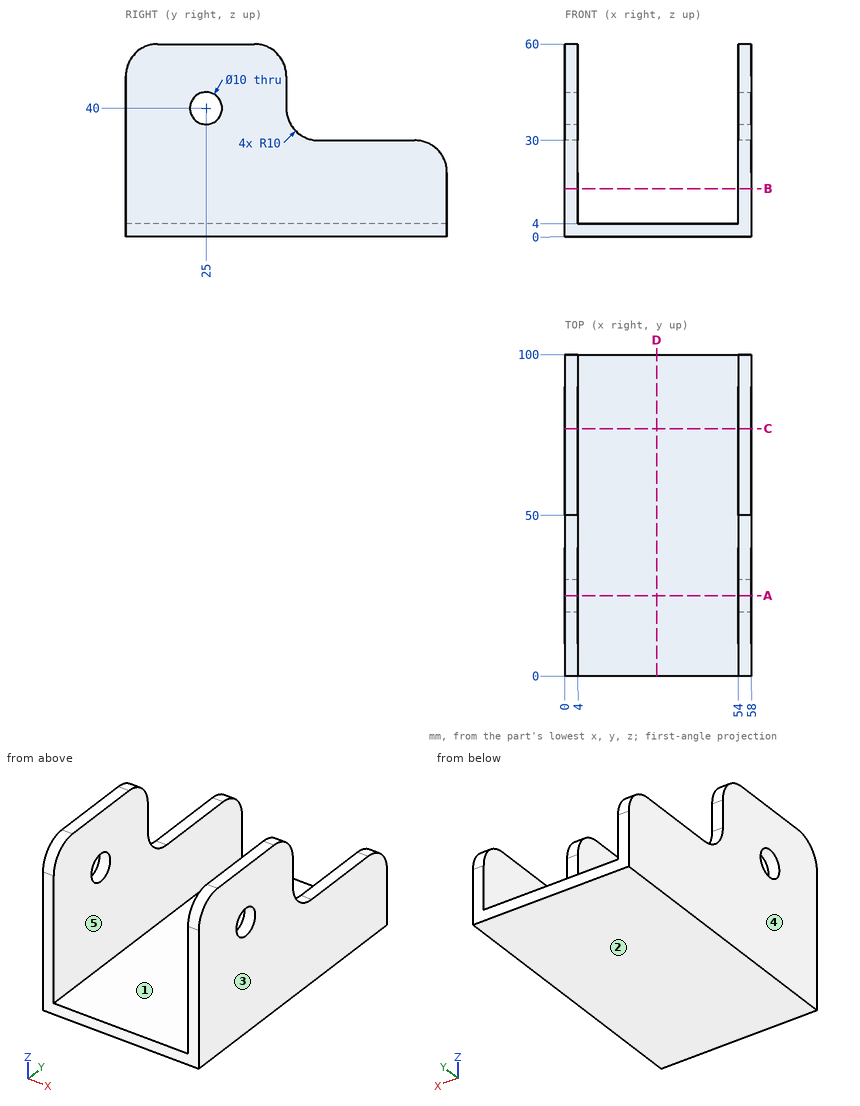
Verification items for this drawing (mm, ordinates from the low corner). A direction names the side the tool comes from. Round coordinates to 2 decimals unless told otherwise and drop trailing zeros. Order: outer loops, then holes, each group sorted by start corner. A loop starts at its lowest first (then second) coordinate and runs counter-clockwise, first axis right, second up. Notation, with made-up numbers: (4.25, 89.25) -> (11.25, 89.25) arc R28 cw to (11.25, 119.25) -> close; hole circle Ø9 at (0, 46). An arc over 180 degrees is marked (long way). Use one line per item in the form item = value.
1. Cross-section at C-C, the plane y = 77. Enter the section's corners in (x, z).
Working result:
outline = (0, 0) -> (58, 0) -> (58, 30) -> (54, 30) -> (54, 4) -> (4, 4) -> (4, 30) -> (0, 30) -> close
2. Scan lines: line 1 along Z through (x, y) = (1, 25); line 2 along X through (y, z) = (80.5, 13.5); line 3 along Z through (x, y) = (2, 67.5). Record each from-to range of solid material in increasing order. Write a range as from..to.
Working result:
line_1 = 0..35, 45..60
line_2 = 0..4, 54..58
line_3 = 0..30
3. Cross-section at D-D, the plane x = 28.5. Enter the section's corners in (y, z).
Working result:
outline = (0, 0) -> (100, 0) -> (100, 4) -> (0, 4) -> close
4. Cross-section at B-B, the plane z = 15. Enter the section's corners in (x, y), plus the area to 3 significant figures.
Working result:
outline = (0, 0) -> (4, 0) -> (4, 100) -> (0, 100) -> close; (54, 0) -> (58, 0) -> (58, 100) -> (54, 100) -> close
area = 800 mm^2
5. Mould release check, pull along X, two halves, no side actions. Record for the marked faces 1, 2 and 3: pulls with the +X half, pulls with the -X half, needs draft (parallel to the pull), parting line crosses it, or undercut.
Working result:
face_1 = undercut
face_2 = needs draft
face_3 = pulls with the +X half
6. Cross-section at A-A, the plane y = 25. Enter the section's corners in (x, z), plus the area to 3 significant figures.
Working result:
outline = (0, 0) -> (58, 0) -> (58, 35) -> (54, 35) -> (54, 4) -> (4, 4) -> (4, 35) -> (0, 35) -> close; (0, 45) -> (4, 45) -> (4, 60) -> (0, 60) -> close; (54, 45) -> (58, 45) -> (58, 60) -> (54, 60) -> close
area = 600 mm^2
7. Go/stop test with flat-tipped pins: pin 1 (4.5 mm diameter, centred on x = 2, y = 80.5, fed in from +Z); pin 2 (11.5 mm diameter, centred on y = 25, z = 40, fed in from +X); pin 3 (1 mm diameter, centred on x = 14, y = 34, fed in from +Z); pin 4 (4.5 mm diameter, centred on x = 56.5, z = 45, fed in from +Y). Record where each tip stops, or that it passes through.
Working result:
pin_1 = 30
pin_2 = 58
pin_3 = 4
pin_4 = 50
8. Set-up check for the marked faces 4 and 5: record each of +Z, -Z, +X, -X, +Y, -Y from which the full face is reachable in a straight line by a thin tool's end or side.
Working result:
face_4 = +Z, -Z, -X, +Y, -Y
face_5 = +Z, +Y, -Y
